Read the model definition and answer for the solid it produces. Units are mm, in the model's axes. A direction names the side the tool comes from. Give positions to 0.01 mm unless a question says otherwise; leave off trailing zeros. Order: outer loops, then holes, each group sorted by start corner. A loop starts at its lowest first (then second) coordinate and runs counter-clockwise, first axis right, second up.
Item 1: Which of the six approach directions +Z, -Z, +X, -X, +Y, -Y give full straight-line access (tool end or side, diameter ignored) to faces 1 (the face through (21.724, 3.219, -16.292)), 2 (the face through (63.5, 3, -36))?
Item 2: A cutting plane is placed at A-A (z = -34). Write down the section's boundary in (x, y).
Item 3: A cutting plane is placed at D-D (x = 38.1). Write down the section's boundary in (y, z), plus the area to 3 significant figures.
Item 4: A cutting plane is placed at C-C (y = 1). Write down the section's boundary in (x, z) (3 decimals).
Item 5: Find the intervals of material crossed by line 1 along X through (y, z) = (2.25, -2.5); line 2 along Z through (x, y) = (39, 3.5); line 3 along X through (y, z) = (5.75, -16.5), in increasing order.
Item 6: The mould has two halves that part along X. Classify faces 3 (the face through (7.7, 3.1, -3.7)), 4 (the face through (52, 0, -29)), 5 (the face through (36, 3, -12.7)), 6 (the face through (0, 3, -3)): +X half, -X half, draft (parallel to the pull), parting line (faces both ways), or undercut.
Item 7: A cutting plane is placed at B-B (x = 10). Write down the section's boundary in (y, z), plus the area to 3 significant figures.
Item 8: Given pin 1 Ø6 at (x, z) = (14, -29) entering from +Y; pin 2 Ø1.5 at (y, z) = (3, -12.5) entering from -X, each flat-ended and moving along its own axis, determine where each tip first touches the part or whether it passes through.
from build123d import *

# Parameters (mm, degrees)
BOSS_EXTRUDE1_DEPTH       = 6.35
F_6_CLEARANCE_HOLE1_D     = 3.7973
F_6_CLEARANCE_HOLE1_DEPTH = 12.7
F_6_CLEARANCE_HOLE1_TIP   = 1.140824014
FILLET1_R                 = 6.35


with BuildPart() as part:
    # Sketch1 → Boss-Extrude1 (new body)
    with BuildSketch(Plane(origin=(0, 0, 0), x_dir=(1, 0, 0), z_dir=(0, 1, 0))):
        Polygon((0, 0), (63.5, 0), (63.5, 73.66), (57.15, 73.66), (0, 6.35), align=None)
        Polygon((13.721627919, 12.7), (50.8, 12.7), (50.8, 56.370082673), align=None, mode=Mode.SUBTRACT)
    extrude(amount=BOSS_EXTRUDE1_DEPTH)

    # #6 Clearance Hole1
    with Locations(Plane(origin=(0, 6.35, 0), x_dir=(1, 0, 0), z_dir=(0, 1, 0))):
        with Locations((9.525, 3.175), (38.1, 3.175), (60.325, 10.16), (60.325, 58.42)):
            Hole(F_6_CLEARANCE_HOLE1_D / 2, depth=F_6_CLEARANCE_HOLE1_DEPTH)
            with Locations((0, 0, -(F_6_CLEARANCE_HOLE1_DEPTH + F_6_CLEARANCE_HOLE1_TIP / 2))):  # 118° drill point
                Cone(0, F_6_CLEARANCE_HOLE1_D / 2, F_6_CLEARANCE_HOLE1_TIP, mode=Mode.SUBTRACT)

    # Fillet1
    fillet1_edges = [part.edges().sort_by_distance(p)[0] for p in [
        (50.8, 3.175, -12.7),
        (50.8, 3.175, -56.370082673),
        (13.721627919, 3.175, -12.7),
    ]]
    fillet(fillet1_edges, radius=FILLET1_R)


solid = part.part
Response values:
1. face 1: +Y, -Y
1. face 2: +Z, -Z, +X, +Y, -Y
2. outline: (23.48, 0) - (31.81, 0) - (31.81, 6.35) - (23.48, 6.35) - close; (50.8, 0) - (63.5, 0) - (63.5, 6.35) - (50.8, 6.35) - close
3. outline: (0, -51.22) - (6.35, -51.22) - (6.35, -41.41) - (0, -41.41) - close; (0, -12.7) - (6.35, -12.7) - (6.35, -5.07) - (0, -5.07) - close; (0, -1.28) - (6.35, -1.28) - (6.35, 0) - (0, 0) - close
3. area: 119 mm2
4. outline: (0, -6.35) - (57.15, -73.66) - (63.5, -73.66) - (63.5, 0) - (0, 0) - close; hole circle Ø3.797 at (9.525, -3.175); hole (22.603, -23.16) - (39.609, -43.19) arc R6.35 ccw to (50.8, -39.08) - (50.8, -19.05) arc R6.35 ccw to (44.45, -12.7) - (27.443, -12.7) arc R6.35 ccw to start; hole circle Ø3.797 at (38.1, -3.175); hole circle Ø3.797 at (60.325, -58.42); hole circle Ø3.797 at (60.325, -10.16)
5. line 1: x = 0 to 7.75, 11.3 to 36.33, 39.87 to 63.5
5. line 2: z = -52.28 to -42.47, -12.7 to -4.85, -1.5 to 0
5. line 3: x = 8.62 to 21.63, 50.27 to 63.5
6. face 3: undercut
6. face 4: draft
6. face 5: undercut
6. face 6: -X half
7. outline: (0, -18.13) - (6.35, -18.13) - (6.35, -5.01) - (0, -5.01) - close; (0, -1.34) - (6.35, -1.34) - (6.35, 0) - (0, 0) - close
7. area: 91.8 mm2
8. pin 1: passes through
8. pin 2: stops at x = 4.58
